```python
from build123d import *

# Parameters (mm, degrees)
F1_DEPTH = 13.462


with BuildPart() as f1:
    # F0 (on Top) → F1 (new body)
    with BuildSketch(Plane.XY):
        with BuildLine():
            ThreePointArc((0, -63.5), (44.901281, -44.901281), (63.5, 0))
            Line((63.5, 0), (4.445, 0))
            ThreePointArc((4.445, 0), (3.14309, -3.14309), (0, -4.445))
            Line((0, -4.445), (0, -63.5))
        make_face()
        with BuildLine():
            ThreePointArc((-63.5, 0), (-44.901281, -44.901281), (0, -63.5))
            Line((0, -63.5), (0, -4.445))
            ThreePointArc((0, -4.445), (-3.14309, -3.14309), (-4.445, 0))
            Line((-4.445, 0), (-63.5, 0))
        make_face()
        with BuildLine():
            Line((4.445, 0), (63.5, 0))
            ThreePointArc((63.5, 0), (44.901281, 44.901281), (0, 63.5))
            Line((0, 63.5), (0, 4.445))
            ThreePointArc((0, 4.445), (3.14309, 3.14309), (4.445, 0))
        make_face()
        with BuildLine():
            Line((0, 4.445), (0, 63.5))
            ThreePointArc((0, 63.5), (-44.901281, 44.901281), (-63.5, 0))
            Line((-63.5, 0), (-4.445, 0))
            ThreePointArc((-4.445, 0), (-3.14309, 3.14309), (0, 4.445))
        make_face()
    extrude(amount=-F1_DEPTH)


solid = f1.part
```
For this review, take the finished solid that the model builds, in its own axes (mm). Give positions to 0.01 mm unless a question says otherwise; leave off trailing zeros. Loops run counter-clockwise (first coordinate to the right, second up) from the corner with the lowest first, then second, coordinate; pieces in that order, holes last. Notation, with made-up numbers: M 43.25,42 L 85.25,42 A14 cw 85.25,47 Z; hole C 0,82 d1. An arc over 180 degrees is marked long. One line per item, written item: value. Start each with the question number.
Q1. Add section C-C (x = 33.5). Give the boundary of the cut face in (y, z).
Q2. Clearance check with flat-ended pins moving along their axes: pin 1 Ø8 at (x, z) = (19, -8) entering from -Y; pin 2 Ø4 at (y, z) = (-27, -3) entering from +X; pin 3 Ø8 at (y, z) = (-15, -10.5) entering from +X. State where each tip first meets the part, or that it passes through.
Q3. Add section A-A (z = -8.5). Give the boundary of the cut face in (x, y) (3 decimals), and give its area (3 significant figures).
Q4. For L1, parallel to Y at x = -0.5, z = -6; L2, parallel to X at y = -4, z = -10; L3, parallel to Y at x = 3, z = -1.25, list the stretches that pass through material, from the lowest coordinate up.
Q5. Add section B-B (y = -2.5). Give the boundary of the cut face in (x, z).
Q6. Add section D-D (y = -24). Give the boundary of the cut face in (x, z), and give its area (3 significant figures).
Reply:
1. outline: M -53.94,-13.46 L 53.94,-13.46 L 53.94,0 L -53.94,0 Z
2. pin 1: y = -61.7
2. pin 2: x = 58.37
2. pin 3: x = 62.54
3. outline: M -63.5,0 A63.5 ccw 0,-63.5 A63.5 ccw 63.5,0 A63.5 ccw 0,63.5 A63.5 ccw Z; hole M -4.445,0 A4.445 ccw 0,-4.445 A4.445 ccw 4.445,0 A4.445 ccw 0,4.445 A4.445 ccw Z
3. area: 12,600 mm²
4. L1: -63.5 to -4.42, 4.42 to 63.5
4. L2: -63.37 to -1.94, 1.94 to 63.37
4. L3: -63.43 to -3.28, 3.28 to 63.43
5. outline: M -63.45,-13.46 L -3.68,-13.46 L -3.68,0 L -63.45,0 Z; M 3.68,-13.46 L 63.45,-13.46 L 63.45,0 L 3.68,0 Z
6. outline: M -58.79,-13.46 L 58.79,-13.46 L 58.79,0 L -58.79,0 Z
6. area: 1,580 mm²
